Part model, mm, in its own coordinate system. Face numbers are marked on the shaded views. Give positions to 0.01 mm unless a question says otherwise; leave off trailing zeros. Write each loop counter-clockwise with the first axis right and the second up, starting at its lowest first coordinate (ties: lowest second). Pieces come first, ordered by that corner, then holes. Notation, with made-up numbers: (88, -40) - (132, -40) arc R23 cw to (132, -4) - close; hole circle Ø10 at (29, -25.75). An arc over 180 degrees is marked (long way). Answer in a Markdown table with one row per item. Add a question column.
1. Band-saw the part on A-A on x = 0. Write the cut outline in (y, z), plus the area to 3 significant figures.
2. Band-saw the part on C-C on z = 8. Write the cut outline in (x, y), plus the area to 3 significant figures.
3. Band-saw the part on B-B on y = -4.75. Write the cut outline in (x, z), plus the area to 3 significant figures.
4. Drop flat-ended pins along their axis: pin 1 Ø1 at (y, z) = (6, 4.5) entering from +X; pin 2 Ø1 at (x, z) = (-10, 8) entering from -Y; pin 3 Ø5 at (x, z) = (5, 9) entering from +Y. Give the stop position or say it passes through.
5. Probe line 1 along Y through (x, z) = (0, 2); line 2 along Y through (x, z) = (0, 9.05); line 3 along Z through (x, y) = (-5.75, -4.5). List the from-to ranges inside material, lowest first.
6. Pull direction Y, two halves, no side cores. Call the marked faces 1, 2 and 3: released by +Y, released by -Y, zero draft, split by the parting line, or undercut.
7. Band-saw the part on D-D on y = 8.5. Write the cut outline in (x, z).
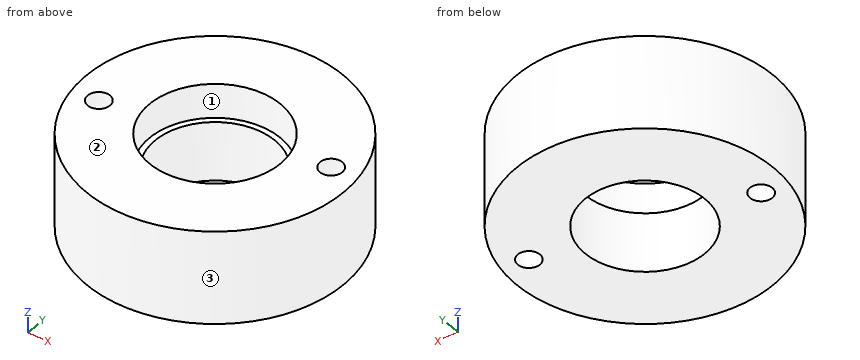
```python
from build123d import *

# Parameters (mm, degrees)
SKETCH_1_R          = 15
SKETCH_1_R_2        = 7
EXTRUDE_1_DEPTH     = 10.9
SKETCH_5_R          = 7.65
CUT_EXTRUDE_3_DEPTH = 4
SKETCH_2_R          = 1.3
CUT_EXTRUDE_4_DEPTH = 24.849737944


with BuildPart() as part:
    # ｽｹｯﾁ1 → ﾎﾞｽ - 押し出し1 (new body)
    with BuildSketch(Plane.XY):
        Circle(SKETCH_1_R)
        Circle(SKETCH_1_R_2, mode=Mode.SUBTRACT)
    extrude(amount=EXTRUDE_1_DEPTH)

    # ｽｹｯﾁ5 → ｶｯﾄ - 押し出し3 (cut)
    with BuildSketch(Plane.XY.offset(10.9)):
        Circle(SKETCH_5_R)
    extrude(amount=-CUT_EXTRUDE_3_DEPTH, mode=Mode.SUBTRACT)

    # ｽｹｯﾁ2 → ｶｯﾄ - 押し出し4 (cut, through all)
    with BuildSketch(Plane(origin=(0, 0, 0), x_dir=(-1, 0, 0), z_dir=(0, 0, -1))):
        with Locations((-11.798830207, 2.188059811)):
            Circle(SKETCH_2_R)
        with Locations((11.798830207, -2.188059811)):
            Circle(SKETCH_2_R)
    extrude(amount=-CUT_EXTRUDE_4_DEPTH, mode=Mode.SUBTRACT)


solid = part.part
```
Values:
| question | item | result |
|---|---|---|
| 1 | outline | (-15, 0) - (-7, 0) - (-7, 6.9) - (-7.65, 6.9) - (-7.65, 10.9) - (-15, 10.9) - close; (7, 0) - (15, 0) - (15, 10.9) - (7.65, 10.9) - (7.65, 6.9) - (7, 6.9) - close |
| 1 | area | 169 mm² |
| 2 | outline | circle Ø30 at (0, 0); hole circle Ø2.6 at (-11.8, -2.19); hole circle Ø15.3 at (0, 0); hole circle Ø2.6 at (11.8, 2.19) |
| 2 | area | 512 mm² |
| 3 | outline | (-14.23, 0) - (-5.14, 0) - (-5.14, 6.9) - (-6, 6.9) - (-6, 10.9) - (-14.23, 10.9) - close; (5.14, 0) - (14.23, 0) - (14.23, 10.9) - (6, 10.9) - (6, 6.9) - (5.14, 6.9) - close |
| 3 | area | 191 mm² |
| 4 | pin 1 | stops at x = 13.96 |
| 4 | pin 2 | stops at y = -11.61 |
| 4 | pin 3 | stops at y = 14.79 |
| 5 | line 1 | y = -15 to -7, 7 to 15 |
| 5 | line 2 | y = -15 to -7.65, 7.65 to 15 |
| 5 | line 3 | z = 0 to 6.9 |
| 6 | face 1 | undercut |
| 6 | face 2 | zero draft |
| 6 | face 3 | split by the parting line |
| 7 | outline | (-12.36, 0) - (12.36, 0) - (12.36, 10.9) - (-12.36, 10.9) - close |
